The figure shows three views and two pictorial views of one solid part (mm, origin at its lowest corner). Answer the questions. Round coordinates to 2 decimals unless told otherwise and drop trailing zeros. Order: outer loops, then holes, each group sorted by start corner. A loop starts at its lowest first (then second) coordinate and runs counter-clockwise, first axis right, second up. Notation, with made-up numbers: M 0.25,85 L 50.25,85 A14 ccw 50.25,99 Z; hole C 83,6 d11. An arc over 180 degrees is marked long. Return JSON: item names as keys, results as strings.
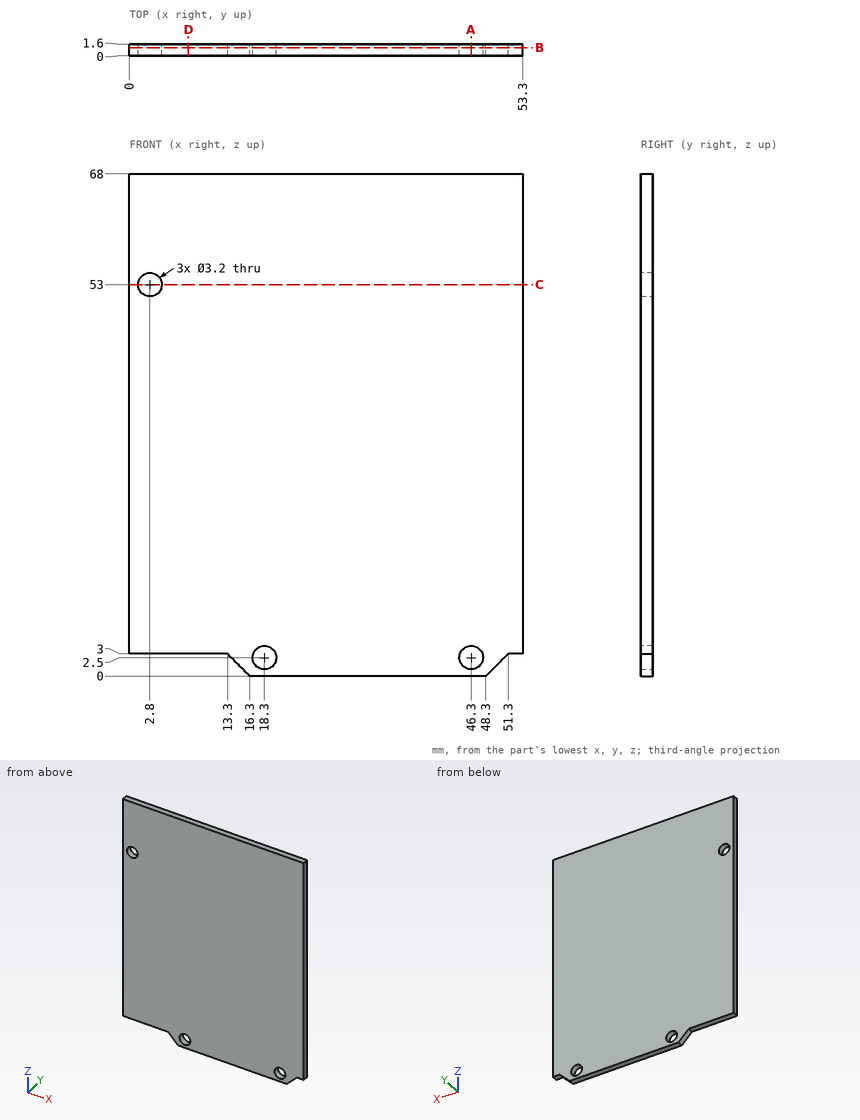
Item 1: Find section A-A (x = 46.3). Determine the outline of the cut face in (y, z), plus the area to 3 significant figures.
Output:
{"outline": "M 0,0 L 1.6,0 L 1.6,0.9 L 0,0.9 Z; M 0,4.1 L 1.6,4.1 L 1.6,68 L 0,68 Z", "area": "104 mm^2"}
Item 2: Consider line 1 along X through (y, z) = (0.8, 2.5); line 2 along Z through (x, y) = (18.5, 1.35); line 3 along X through (y, z) = (0.75, 53). Determine where each line is inside the solid, lowest interval first. Write a range as [from, to].
Output:
{"line 1": "x = [13.8, 16.7], [19.9, 44.7], [47.9, 50.8]", "line 2": "z = [0, 0.91], [4.09, 68]", "line 3": "x = [0, 1.2], [4.4, 53.3]"}
Item 3: Each of these flat-tipped pins is pushed along its axis until it touches: pin 1 (2 mm diameter, centred on x = 28.5, z = 58, fed in from -Y); pin 2 (2.5 mm diameter, centred on x = 46.3, z = 2.5, fed in from +Y). Where does it stop, or does it pass through?
Output:
{"pin 1": "stops at y = 0", "pin 2": "passes through"}
Item 4: Find section D-D (x = 8). Determine the outline of the cut face in (y, z).
Output:
{"outline": "M 0,3 L 1.6,3 L 1.6,68 L 0,68 Z"}
Item 5: Find section B-B (y = 1.1). Determine the outline of the cut face in (x, z), plus the area to 3 significant figures.
Output:
{"outline": "M 0,3 L 13.3,3 L 16.3,0 L 48.3,0 L 51.3,3 L 53.3,3 L 53.3,68 L 0,68 Z; hole C 2.8,53 d3.2; hole C 18.3,2.5 d3.2; hole C 46.3,2.5 d3.2", "area": "3,550 mm^2"}
Item 6: Find section C-C (z = 53). Determine the outline of the cut face in (x, y).
Output:
{"outline": "M 0,0 L 1.2,0 L 1.2,1.6 L 0,1.6 Z; M 4.4,0 L 53.3,0 L 53.3,1.6 L 4.4,1.6 Z"}
